CAD build for the part. Positions are in the model's coordinates, mm. A direction names the side the tool comes from. Give positions to 0.01 mm unless a question says otherwise; leave off trailing zeros. Write each loop counter-clockwise with the first axis right and the second up, starting at its lowest first coordinate (ties: lowest second). Pieces come first, ordered by that corner, then holes. Notation, with made-up numbers: (86, 42) -> (127, 42) arc R15 cw to (127, 54) -> close; hole circle Ø7 at (8.25, 30). An arc over 180 degrees is marked (long way). Answer as a JSON object with one key per item and string values.
```python
from build123d import *

# Parameters (mm, degrees)
BOSS_EXTRUDE1_DEPTH     = 6.35
CUT_EXTRUDE3_DEPTH      = 40.185503571
CUT_EXTRUDE3_DEPTH_BACK = 40.185503571
SKETCH2_R               = 1.55
BOSS_EXTRUDE2_DEPTH     = 6.35
FILLET1_R               = 2


with BuildPart() as part:
    # Sketch1 → Boss-Extrude1 (new body)
    with BuildSketch(Plane.XY):
        Polygon((24, -4), (16, -15), (-24, -28.159033899), (-26.5, -20.559691822), (10, -10), (14, -4), (-24, -4), (-24, 4), (24, 4), align=None)
    extrude(amount=BOSS_EXTRUDE1_DEPTH)

    # Sketch2 → Cut-Extrude3 (cut, two sides: drawn at the far end of the back side and taken through both)
    with BuildSketch(Plane.XY.offset(-CUT_EXTRUDE3_DEPTH_BACK)):
        with Locations((-19, 0)):
            Circle(SKETCH2_R)
        with Locations((17, 0)):
            Circle(SKETCH2_R)
        with Locations((-22, -22.901341131)):
            Circle(SKETCH2_R)
    extrude(amount=CUT_EXTRUDE3_DEPTH + CUT_EXTRUDE3_DEPTH_BACK, mode=Mode.SUBTRACT)

    # Sketch3 → Boss-Extrude2 (add)
    with BuildSketch(Plane.XY.offset(6.35)):
        Polygon((-12.416374587, -4), (14, -4), (10, -10), (-15.342860583, -17.33185747), (-2.958518174, -8.617728358), align=None)
    extrude(amount=-BOSS_EXTRUDE2_DEPTH)

    # Fillet1
    fillet1_edges = [part.edges().sort_by_distance(p)[0] for p in [
        (24, -4, 3.175),
        (16, -15, 3.175),
        (-24, -28.159033899, 3.175),
        (-26.5, -20.559691822, 3.175),
        (-24, -4, 3.175),
        (-24, 4, 3.175),
        (24, 4, 3.175),
        (-2.958518174, -8.617728358, 3.175),
    ]]
    fillet(fillet1_edges, radius=FILLET1_R)


solid = part.part
```
1) Slice it at C-C (z = 3.5). List the corners of the cut face in (x, y) (3 decimals), then the cut area to 3 significant figures.
Model answer:
{"outline": "(-25.852, -22.53) -> (-24.625, -26.259) arc R2 ccw to (-22.1, -27.534) -> (15.387, -15.202) arc R2 ccw to (16.38, -14.478) -> (23.617, -4.526) arc R2 ccw to (24, -3.35) -> (24, 2) arc R2 ccw to (22, 4) -> (-22, 4) arc R2 ccw to (-24, 2) -> (-24, -2) arc R2 ccw to (-22, -4) -> (-12.416, -4) -> (-6, -7.133) arc R2 cw to (-5.727, -10.566) -> (-15.343, -17.332) -> (-24.508, -19.983) arc R2 ccw to start; hole circle Ø3.1 at (-22, -22.901); hole circle Ø3.1 at (-19, 0); hole circle Ø3.1 at (17, 0)", "area": "902 mm2"}
2) Slice it at D-D (y = -12). List the corners of the cut face in (x, z).
Model answer:
{"outline": "(-7.77, 0) -> (18.18, 0) -> (18.18, 6.35) -> (-7.77, 6.35) -> close"}
3) Slice it at B-B (x = 17). List the corners of the cut face in (y, z) (3 decimals).
Model answer:
{"outline": "(-13.625, 0) -> (-1.55, 0) -> (-1.55, 6.35) -> (-13.625, 6.35) -> close; (1.55, 0) -> (4, 0) -> (4, 6.35) -> (1.55, 6.35) -> close"}
4) Wall check: probe 1 along X at (y, z) = (0, 4); probe 2 along Y at (x, z) = (-19, 2.5); probe 3 along Y at (x, z) = (17, 4.5) (3 decimals). Give the ranges that are in metal, low to high.
Model answer:
{"probe 1": "x = -24 to -20.55, -17.45 to 15.45, 18.55 to 24", "probe 2": "y = -26.51 to -18.39, -4 to -1.55, 1.55 to 4", "probe 3": "y = -13.625 to -1.55, 1.55 to 4"}
5) Slice it at A-A (y = 0.5). List the corners of the cut face in (x, z), then the cut area to 3 significant figures.
Model answer:
{"outline": "(-24, 0) -> (-20.47, 0) -> (-20.47, 6.35) -> (-24, 6.35) -> close; (-17.53, 0) -> (15.53, 0) -> (15.53, 6.35) -> (-17.53, 6.35) -> close; (18.47, 0) -> (24, 0) -> (24, 6.35) -> (18.47, 6.35) -> close", "area": "268 mm2"}
6) Mould opens along Y. For faces 4 (the flat face through (-1, -8, 0)), 5 (the cylindrical face through (15.45, 0.07, 3.13)), 6 (the cylindrical face through (-23.646, -27.41, 3.219)), 7 (the cylindrical face through (-4.88, -8.8, 3.13)) say: released by +Y, released by -Y, zero draft, split by the parting line, or undercut.
Model answer:
{"face 4": "zero draft", "face 5": "undercut", "face 6": "released by -Y", "face 7": "undercut"}
7) 3-axis set-ups, long thin cutter, end or side, ignore diameter. For faces 1 (the cylindrical face through (-23.4, -3.43, 3.22)), 2 (the flat face through (-24, 0, 3)), 3 (the cylindrical face through (23.43, 3.4, 3.22)): which of +Z, -Z, +X, -X, +Y, -Y reach the whole face in a straight line?
Model answer:
{"face 1": "+Z, -Z, -X", "face 2": "+Z, -Z, -X, +Y", "face 3": "+Z, -Z, +X, +Y"}
8) Pin check, flat tip, straight feed: pin 1 (1 mm diameter, centred on y = -13, z = 1.5, fed in from -X). Stop position of the tip, or through.
Model answer:
{"pin 1": "stops at x = -9.9"}
